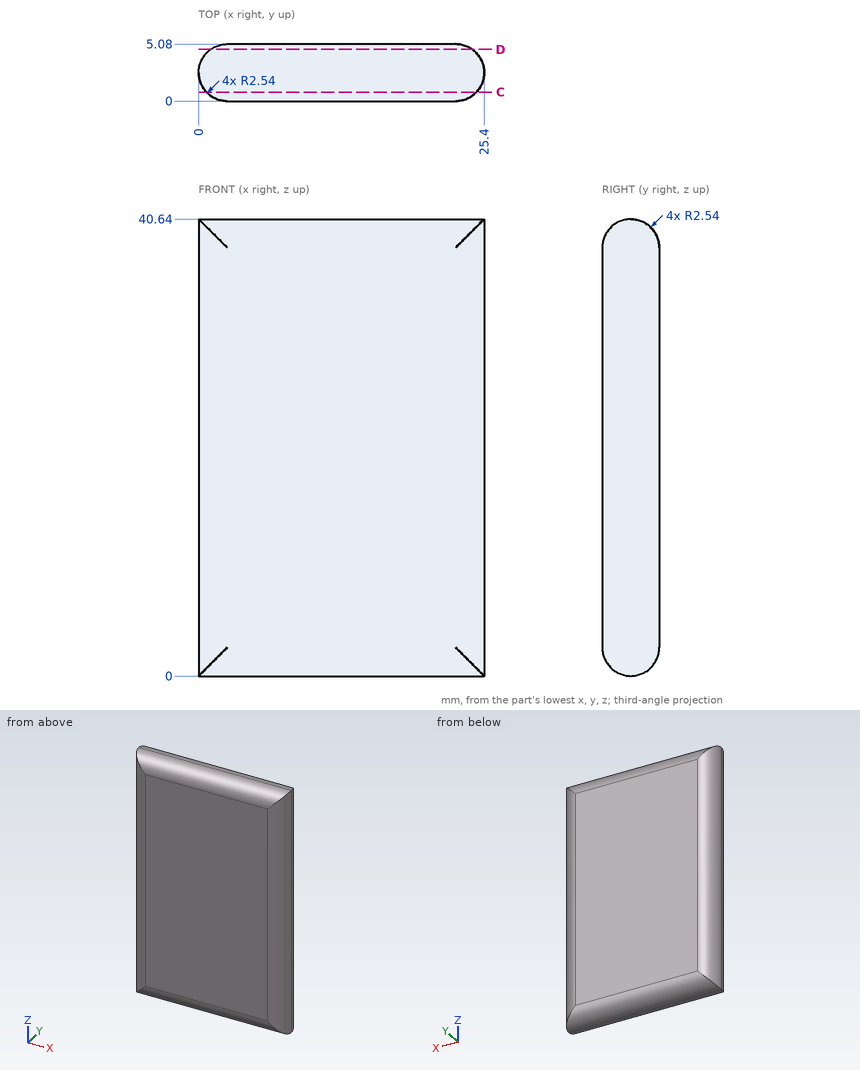
Here's the drawing with two shaded views (mm, measured from the low corner). I have some questions. Give positions to 0.01 mm unless a question says otherwise; leave off trailing zeros. Loops run counter-clockwise (first coordinate to the right, second up) from the corner with the lowest first, then second, coordinate; pieces in that order, holes last. Notation, with made-up numbers: (70, 85.25) -> (122, 85.25) arc R25 cw to (122, 117.25) -> close; hole circle Ø3 at (84.5, 87). An arc over 180 degrees is marked (long way). Answer as a JSON object with one key per item and string values. Group by question number.
Item 1: Imagine slicing it at C-C on y = 0.8. Write out the boundary of the cut face in (x, z), then the cut area to 3 significant figures.
Item 2: Imagine slicing it at D-D on y = 4.6. Write out the boundary of the cut face in (x, z).
Item 3: I need wall thicknesses on L1, parallel to X at y = 2.75, z = 37.5; L2, parallel to Z at x = 7.25, y = 2.3; L3, parallel to X at y = 1.6, z = 20. Which ranges of each line are inside material? Lowest first, please.
Item 4: Will this pin go through, and if not, where does the flat tip stop? pin 1 (1 mm diameter, centred on x = 3.5, y = 3.5, fed in from -Z).
Answer list:
{
 "1": {"outline": "(0.69, 0.69) -> (24.71, 0.69) -> (24.71, 39.95) -> (0.69, 39.95) -> close", "area": "943 mm2"},
 "2": {"outline": "(1.05, 1.05) -> (24.35, 1.05) -> (24.35, 39.59) -> (1.05, 39.59) -> close"},
 "3": {"L1": "x = 0.01 to 25.39", "L2": "z = 0.01 to 40.63", "L3": "x = 0.18 to 25.22"},
 "4": {"pin 1": "stops at z = 0.04"}
}
